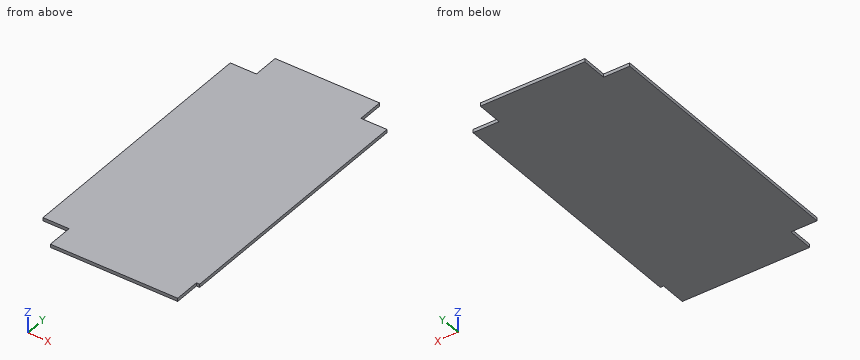
Autodesk Fusion 360 part; units mm, degrees
sketch "Sketch1" plane through (0, 0, 0) normal (0, 0, 1) x (1, 0, 0)
  line L0 (0, 0) -> (0, 609.6)
  line L1 (0, 609.6) -> (304.8, 609.6)
  line L2 (304.8, 609.6) -> (304.8, 0)
  line L3 (304.8, 0) -> (0, 0)
  line L4 (0, 0) -> (50.8, 0)
  line L5 (50.8, 0) -> (50.8, 50.8)
  line L6 (50.8, 50.8) -> (0, 50.8)
  line L7 (0, 50.8) -> (0, 0)
  line L8 (0, 609.6) -> (50.8, 609.6)
  line L9 (50.8, 609.6) -> (50.8, 558.8)
  line L10 (50.8, 558.8) -> (0, 558.8)
  line L11 (0, 558.8) -> (0, 609.6)
  line L12 (304.8, 609.6) -> (254, 609.6)
  line L13 (254, 609.6) -> (254, 558.8)
  line L14 (254, 558.8) -> (304.8, 558.8)
  line L15 (304.8, 558.8) -> (304.8, 609.6)
  line L16 (304.8, 0) -> (298.45, 0)
  line L17 (298.45, 0) -> (298.45, 50.8)
  line L18 (298.45, 50.8) -> (304.8, 50.8)
  line L19 (304.8, 50.8) -> (304.8, 0)
  dimension "d2" = 609.6
  dimension "d3" = 304.8
  dimension "d10" = 50.8
  dimension "d11" = 50.8
  dimension "d12" = 50.8
  dimension "d13" = 50.8
  dimension "d14" = 6.35
  dimension "d16" = 304.8
extrude "Extrude1" add sketch "Sketch1" along normal blind 6.35 contours L0 L1 L2 L3 L5 L6 L9 L10 L13 L14 L17 L18
Design review of the part built by this model. Coordinates are the model's own, in mm. Coordinates: 2 decimals unless noted, no trailing zeros. Loops run counter-clockwise (first coordinate to the right, second up) from the corner with the lowest first, then second, coordinate; pieces in that order, holes last. Notation, with made-up numbers: (55.25, 5.25) - (79.25, 5.25) arc R25 cw to (79.25, 31.25) - close; hole circle Ø1 at (-28, 12). An arc over 180 degrees is marked (long way). Use CSV: the item, a comma, the result in double quotes. Start each with the question number.
1) Consider section A-A on z = 1.5. Write out the cut boundary in (x, y).
2) Wall thickness on L1, parallel to X at y = 576.5, z = 0.5; L2, parallel to Y at x = 41, z = 2.75; L3, parallel to X at y = 38.5, z = 3: over which ranges is each line inside the solid? List them lowest first. Write a range as from..to.
3) Consider section C-C on y = 42. Write out the cut boundary in (x, z), then the cut area to 3 significant figures.
4) For pin 1 Ø1.9 at (x, z) = (283, 3) entering from +Y; pin 2 Ø3 at (y, z) = (65.5, 1.5) entering from -X; pin 3 Ø3 at (y, z) = (582.5, 2) entering from -X, all flat-tipped, find the tip position at first contact; note any pin that passes through.
5) Consider section B-B on x = 272. Write out the cut boundary in (y, z), then the cut area to 3 significant figures.
Geometry says:
1,outline,"(0, 50.8) - (50.8, 50.8) - (50.8, 0) - (298.45, 0) - (298.45, 50.8) - (304.8, 50.8) - (304.8, 558.8) - (254, 558.8) - (254, 609.6) - (50.8, 609.6) - (50.8, 558.8) - (0, 558.8) - close"
2,L1,"50.8..254"
2,L2,"50.8..558.8"
2,L3,"50.8..298.45"
3,outline,"(50.8, 0) - (298.45, 0) - (298.45, 6.35) - (50.8, 6.35) - close"
3,area,"1,570 mm^2"
4,pin 1,"y = 558.8"
4,pin 2,"x = 0"
4,pin 3,"x = 50.8"
5,outline,"(0, 0) - (558.8, 0) - (558.8, 6.35) - (0, 6.35) - close"
5,area,"3,550 mm^2"
